```python
from build123d import *

# Parameters (mm, degrees)
F1_DEPTH      = 12.7
F5_DEPTH      = 511.1661396565
F5_DEPTH_BACK = 511.1661396565
F7_DEPTH      = 457.201


with BuildPart() as f1:
    # F0 (on Front) → F1 (new body)
    with BuildSketch(Plane.XZ):
        Polygon((0, -457.2), (0, 0), (-914.4, 0), align=None)
    extrude(amount=F1_DEPTH)

    # F4 (on line) → F5 (cut, two sides)
    with BuildSketch(Plane(origin=(-274.32, 0, 137.16), x_dir=(0, 1, 0), z_dir=(0.894427191, 0, -0.4472135955))) as f5_sk:
        Polygon((-12.7, -408.9321117252), (0, -408.9321117252), (0, -406.8387485734), align=None)
    extrude(amount=-F5_DEPTH, mode=Mode.SUBTRACT)
    extrude(f5_sk.sketch, amount=F5_DEPTH_BACK, mode=Mode.SUBTRACT)

    # F6 (on face) → F7 (cut, through all)
    with BuildSketch(Plane.XY):
        Polygon((-912.0595488455, -6.35), (-810.468111026, -6.35), (-808.223047, 0), (-909.719097691, 0), align=None)
        Polygon((-812.7131750519, -12.7), (-810.468111026, -6.35), (-912.0595488455, -6.35), (-914.4, -12.7), align=None)
        Polygon((-2.245064026, -6.35), (0, -6.35), (0, 0), align=None)
        Polygon((0, -12.7), (0, -6.35), (-2.245064026, -6.35), (-4.4901280519, -12.7), align=None)
    extrude(amount=-F7_DEPTH, mode=Mode.SUBTRACT)


solid = f1.part
```
The listing builds one solid part. Answer for the finished solid, in the listing's coordinates (mm). Coordinates: 2 decimals unless noted, no trailing zeros. Write each loop counter-clockwise with the first axis right and the second up, starting at its lowest first coordinate (ties: lowest second). Pieces come first, ordered by that corner, then holes. Notation, with made-up numbers: (-3, 46) - (21, 46) arc R21 ccw to (21, 78) - close; hole circle Ø10 at (-38.75, 2.25). An arc over 180 degrees is marked (long way). Return JSON: item names as keys, results as strings. Group by question number.
1. Straight lines are drawn through the part: L1, parallel to Z at x = -62.5, y = -8.5; L2, parallel to X at y = -6, z = -401; L3, parallel to Z at x = -451, y = -10. For each, find the intervals that lie inside material, in ascending order.
2. A cutting plane is placed at D-D, the plane z = -153.5. Determine the outline of the cut face in (x, y).
3. A cutting plane is placed at C-C, the plane x = -104.5. Determine the outline of the cut face in (y, z), plus the area to 3 significant figures.
4. Given pin 1 (3 mm diameter, centred on x = -407, z = -55.5, fed in from +Y); pin 2 (4 mm diameter, centred on y = -1.5, z = -256, fed in from -X); pin 3 (1 mm diameter, centred on x = -264, y = -5.5, fed in from -Z), each flat-ended and moving along its own axis, determine where each tip first touches the part or whether it passes through.
5. A cutting plane is placed at A-A, the plane z = -369.5. Determine the outline of the cut face in (x, y).
6. A cutting plane is placed at B-B, the plane y = -3. Determine the outline of the cut face in (x, z).
Ans:
{
 "1": {"L1": "-425.18 to 0", "L2": "-109.93 to -2.12", "L3": "-231.2 to 0"},
 "2": {"outline": "(-607.4, -12.7) - (-4.49, -12.7) - (0, 0) - (-602.72, 0) - close"},
 "3": {"outline": "(-12.7, -404.95) - (0, -402.61) - (0, 0) - (-12.7, 0) - close", "area": "5,130 mm²"},
 "4": {"pin 1": "y = 0", "pin 2": "x = -402.34", "pin 3": "z = -324.14"},
 "5": {"outline": "(-175.4, -12.7) - (-4.49, -12.7) - (0, 0) - (-170.72, 0) - close"},
 "6": {"outline": "(-809.28, -50.77) - (-1.06, -454.88) - (-1.06, 0) - (-809.28, 0) - close"}
}
